Read the model definition and answer for the solid it produces. Units are mm, in the model's axes. Face numbers are marked on the shaded views. A direction names the side the tool comes from. Round coordinates to 2 decimals unless told otherwise and drop trailing zeros. Order: outer loops, then holes, each group sorted by start corner. A loop starts at its lowest first (then second) coordinate and runs counter-clockwise, first axis right, second up. Notation, with made-up numbers: (-12.5, 50) - (10.5, 50) arc R31 ccw to (10.5, 83) - close; hole circle Ø3 at (88.5, 61.25). An arc over 180 degrees is marked (long way). One line per question, with ' | ' between items. Start each with the question number.
1) Straight lines are drawn through the part: line 1 (Y direction, x = -6.25, z = -1.5); line 2 (Y direction, x = 1, z = -19); line 3 (Z direction, x = -7.75, y = 25). For each, find the intervals that lie inside material, in ascending order. Write a range as from..to.
2) The part is cut by section D-D, the plane y = -19. Give the vertices of the cut face in (x, z).
3) The part is cut by section B-B, the plane z = -9. Give the vertices of the cut face in (x, y).
4) The part is cut by section C-C, the plane z = -18.5. Give the vertices of the cut face in (x, y).
5) For the marked faces 5 and 6, determine the directions among +Z, -Z, +X, -X, +Y, -Y from which every point of the face is accessible in a straight line to the end or side of a thin tool.
6) Flat-ended cylindrical pins translate along their axes: pin 1 (1 mm diameter, centred on x = -1.5, z = -3.5, fed in from +Y); pin 2 (3 mm diameter, centred on x = -3, y = 5.5, fed in from -Z); pin 3 (1 mm diameter, centred on x = -4, z = -35.5, fed in from -Y) (3 decimals). Find the tip coordinate at first contact, or state that the pin passes through.
7) The mould has two halves that part along Y. Classify the marked faces 1, 2, 3 and 4: pulls with the +Y half, pulls with the -Y half, needs draft (parallel to the pull), parting line crosses it, or undercut.
8) The part is cut by section A-A, the plane y = -26. Give the vertices of the cut face in (x, z), plus the area to 3 significant figures.
from build123d import *

# Parameters (mm, degrees)
PAD_DEPTH            = 10
POCKET004_DEPTH      = 10.001
POCKET004_DEPTH_BACK = 10.001
FILLET_R             = 5


with BuildPart() as part:
    # Sketch031 → Pad (new body, symmetric)
    with BuildSketch(Plane.YZ):
        with BuildLine():
            ThreePointArc((-25.1785714286, 6.0873812391), (-20.8275502166, -31.8153069654), (17.2072930905, -34.7978986763))
            ThreePointArc((19.0972829456, -33.698609943), (18.1291736499, -34.2085141395), (17.2072930905, -34.7978986763))
            ThreePointArc((19.0972829456, -33.698609943), (22.5681914002, -31.4789887478), (25.3748102311, -28.4628961617))
            ThreePointArc((25.3748102311, -28.4628961617), (31.145297274, -12.7793024717), (28.0089705885, 3.6352364091))
            ThreePointArc((28.2330423532, 3.7461049992), (28.0655721758, 3.8027065865), (28.0089705885, 3.6352364091))
            ThreePointArc((31.066665528, -15.4302839547), (31.1616320501, -5.6186996886), (28.2330423532, 3.7461049992))
            Line((31.066665528, -15.4302839547), (32.0529088781, -15.595583847))
            ThreePointArc((32.0529088781, -15.595583847), (32.1508902105, -5.4725207152), (29.129329412, 4.1895793594))
            ThreePointArc((29.129329412, 4.1895793594), (27.6220978156, 4.6989936454), (27.1126835297, 3.1917620489))
            ThreePointArc((24.5628424703, -27.8791938768), (30.1486495946, -12.6974892471), (27.1126835297, 3.1917620489))
            ThreePointArc((18.6688560963, -32.7950334743), (21.9277036404, -30.7110203695), (24.5628424703, -27.8791938768))
            ThreePointArc((18.6688560963, -32.7950334743), (17.6263968436, -33.3440978723), (16.6337166542, -33.978746632))
            ThreePointArc((-24.3392857143, 5.5436906196), (-20.1332985427, -31.0955746448), (16.6337166542, -33.978746632))
            ThreePointArc((-22.6352951412, 5.5022803073), (-23.4757052121, 5.9997048381), (-24.3392857143, 5.5436906196))
            ThreePointArc((-22.6352951412, 5.5022803073), (-20.1217753495, 2.7817742688), (-16.6898993292, 1.3885184309))
            ThreePointArc((-16.6898993292, 1.3885184309), (0, 0), (16.6898993292, 1.3885184309))
            ThreePointArc((16.6898993292, 1.3885184309), (20.1217753495, 2.7817742688), (22.6352951412, 5.5022803073))
            ThreePointArc((24.3392857143, 5.5436906196), (23.4757052121, 5.9997048381), (22.6352951412, 5.5022803073))
            ThreePointArc((27.2641709757, -0.3407779116), (25.9689416046, 2.6845699939), (24.3392857143, 5.5436906196))
            ThreePointArc((27.2641709757, -0.3407779116), (26.9390804209, -1.6832404813), (27.0677858666, -3.0584948317))
            ThreePointArc((22.1178198442, -27.393137735), (27.4381060497, -15.80458599), (27.0677858666, -3.0584948317))
            ThreePointArc((22.1178198442, -27.393137735), (22.2945348248, -28.7962670289), (23.6976641188, -28.6195520483))
            ThreePointArc((23.6976641188, -28.6195520483), (29.9727276849, -11.5022412242), (25.1785714286, 6.0873812391))
            ThreePointArc((25.1785714286, 6.0873812391), (23.4514104243, 6.9994096762), (21.7705902823, 6.0045606146))
            ThreePointArc((16.5246528012, 2.3747707237), (19.5527787015, 3.6041141101), (21.7705902823, 6.0045606146))
            ThreePointArc((-16.5246528012, 2.3747707237), (0, 1), (16.5246528012, 2.3747707237))
            ThreePointArc((-21.7705902823, 6.0045606146), (-19.5527787015, 3.6041141101), (-16.5246528012, 2.3747707237))
            ThreePointArc((-21.7705902823, 6.0045606146), (-23.4514104243, 6.9994096762), (-25.1785714286, 6.0873812391))
        make_face()
        Polygon((27.5840933648, -3.4048594066), (28.2878580479, -7.5454771468), (29.4708916879, -7.3444015231), (28.7671270049, -3.2037837828), align=None, mode=Mode.SUBTRACT)
        Polygon((27.5163556374, -17.3102281064), (26.1710903804, -21.2889542076), (27.3078692665, -21.6733157096), (28.6531345235, -17.6945896084), align=None, mode=Mode.SUBTRACT)
    extrude(amount=PAD_DEPTH, both=True)

    # Sketch039 → Pocket004 (cut, two sides)
    with BuildSketch(Plane.YZ) as pocket004_sk:
        with BuildLine():
            Line((27.4949433361, -3.1040168152), (28.2442255017, -7.2366402237))
            ThreePointArc((28.2442255017, -7.2366402237), (28.4905833373, -7.7742998522), (28.964758919, -8.1277508063))
            ThreePointArc((28.3448300239, -16.5415137543), (28.9619594976, -12.3572643032), (28.964758919, -8.1277508063))
            ThreePointArc((28.3448300239, -16.5415137543), (27.8239715042, -16.8216502598), (27.501471991, -17.3173962868))
            Line((26.1545833247, -21.2955731206), (27.501471991, -17.3173962868))
            ThreePointArc((26.1545833247, -21.2955731206), (26.1095843724, -21.8852723266), (26.3531287482, -22.4242122085))
            ThreePointArc((23.1927484305, -27.7003268604), (24.9130052946, -25.1461691628), (26.3531287482, -22.4242122085))
            Line((23.1927484305, -27.7003268604), (23.2721556366, -27.7601644822))
            ThreePointArc((23.2721556366, -27.7601644822), (25.001049311, -25.1926749171), (26.4478472443, -22.4562809862))
            ThreePointArc((26.4478472443, -22.4562809862), (26.968705764, -22.1761444807), (27.2912052772, -21.6803984538))
            Line((28.6380939435, -17.70222162), (27.2912052772, -21.6803984538))
            ThreePointArc((28.6380939435, -17.70222162), (28.6830928958, -17.112522414), (28.43954852, -16.5735825321))
            ThreePointArc((28.43954852, -16.5735825321), (29.0611192972, -12.3645704307), (29.0631547145, -8.1099107548))
            ThreePointArc((29.0631547145, -8.1099107548), (29.3830587907, -7.6124859451), (29.424975047, -7.022559605))
            Line((29.424975047, -7.022559605), (28.6756928814, -2.8899361965))
            ThreePointArc((28.6756928814, -2.8899361965), (28.4127513004, -2.3450081602), (27.9069175932, -2.0130185515))
            ThreePointArc((27.9069175932, -2.0130185515), (27.5498359522, -2.5014625518), (27.4949433361, -3.1040168152))
        make_face()
    extrude(amount=-POCKET004_DEPTH, mode=Mode.SUBTRACT)
    extrude(pocket004_sk.sketch, amount=POCKET004_DEPTH_BACK, mode=Mode.SUBTRACT)

    # Fillet
    fillet_edges = [part.edges().sort_by_distance(p)[0] for p in [
        (10, 31.559787, -15.512934),
        (-10, 31.559787, -15.512934),
    ]]
    fillet(fillet_edges, radius=FILLET_R)


solid = part.part
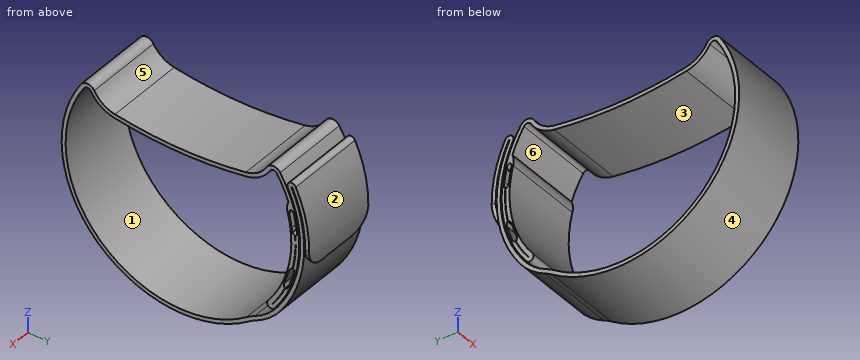
Values:
1) line 1: y = -28.7..-27.66, 26.96..28.7, 28.96..30.01, 30.27..31.31 | line 2: y = -28.69..-27.64, 26.59..26.93, 28.21..28.69, 28.95..29.99 | line 3: z = -28.96..-27.25, -26.81..-25.19, -25..-22.83, 4.47..6.32
2) outline: (-10, -33.44) - (10, -33.44) - (10, -32.13) - (-10, -32.13) - close; (-10, 2.13) - (10, 2.13) - (10, 3.26) - (-10, 3.26) - close
3) outline: (-10, -29.98) - (10, -29.98) - (10, -28.97) - (-10, -28.97) - close; (-10, 27.97) - (10, 27.97) - (10, 29.01) - (-10, 29.01) - close; (-10, 29.11) - (10, 29.11) - (10, 29.98) - (-10, 29.98) - close; (-10, 30.23) - (10, 30.23) - (10, 31.23) - (-10, 31.23) - close; (-10, 31.48) - (10, 31.48) - (10, 32.48) - (-10, 32.48) - close
4) outline: (-10, -28.84) - (10, -28.84) - (10, -27.79) - (-10, -27.79) - close; (-10, 26.75) - (10, 26.75) - (10, 27.1) - (-10, 27.1) - close; (-10, 28.38) - (10, 28.38) - (10, 28.84) - (-10, 28.84) - close; (-10, 29.1) - (10, 29.1) - (10, 30.13) - (-10, 30.13) - close
5) face 5: +Z, +X, -X | face 6: +X, -X
6) pin 1: stops at y = 31.9 | pin 2: stops at z = -39.96 | pin 3: stops at y = -16.915
7) face 1: undercut | face 2: pulls with the +Y half | face 3: undercut | face 4: parting line crosses it
8) outline: (-10, -25.19) - (10, -25.19) - (10, -23.07) - (-10, -23.07) - close; (-10, 2.62) - (10, 2.62) - (10, 4.74) - (-10, 4.74) - close | area: 84.9 mm^2
